from build123d import *

# Parameters (mm, degrees)
BOSS_EXTRUDE1_DEPTH = 2.5
SKETCH2_R           = 2
SKETCH2_R_2         = 1
CUT_EXTRUDE1_DEPTH  = 5
BOSS_EXTRUDE2_DEPTH = 13
SKETCH6_W           = 75
SKETCH6_H           = 9
BOSS_EXTRUDE3_DEPTH = 7
BOSS_EXTRUDE4_DEPTH = 10
SKETCH8_W           = 38.5
SKETCH8_H           = 0.01
BOSS_EXTRUDE5_DEPTH = 0.3


with BuildPart() as part:
    # Sketch1 → Boss-Extrude1 (new body)
    with BuildSketch(Plane(origin=(0, 0, 0), x_dir=(1, 0, 0), z_dir=(0, 1, 0))):
        with BuildLine():
            Line((-58.5, 47.5), (58.5, 47.5))
            Line((58.5, 47.5), (58.5, 25))
            ThreePointArc((58.5, 25), (56, 22.5), (58.5, 20))
            Line((58.5, 20), (58.5, -47.5))
            Line((58.5, -47.5), (-52.5, -47.5))
            Line((-52.5, -47.5), (-52.5, -2.5))
            Line((-52.5, -2.5), (-58.5, 5.5))
            Line((-58.5, 5.5), (-58.5, 20))
            ThreePointArc((-58.5, 20), (-56, 22.5), (-58.5, 25))
            Line((-58.5, 25), (-58.5, 47.5))
        make_face()
    extrude(amount=BOSS_EXTRUDE1_DEPTH)

    # Sketch2 → Cut-Extrude1 (cut)
    with BuildSketch(Plane(origin=(0, 2.5, 0), x_dir=(1, 0, 0), z_dir=(0, 1, 0))):
        with Locations(Location((-11.054054054, 6.409494198, 0), (0, 0, 270))):
            Circle(SKETCH2_R)
        with Locations(Location((-30, -32.5, 0), (0, 0, 270))):
            Circle(SKETCH2_R)
        with Locations(Location((38.5, -32.5, 0), (0, 0, 270))):
            Circle(SKETCH2_R)
        with Locations(Location((-42.5, -45.5, 0), (0, 0, 270))):
            Circle(SKETCH2_R_2)
        with Locations(Location((31.5, -45.5, 0), (0, 0, 270))):
            Circle(SKETCH2_R_2)
    extrude(amount=-CUT_EXTRUDE1_DEPTH, mode=Mode.SUBTRACT)

    # Sketch3 → Boss-Extrude2 (add)
    with BuildSketch(Plane(origin=(0, 2.5, 0), x_dir=(1, 0, 0), z_dir=(0, 1, 0))):
        Polygon((-26.5, 47.5), (-26.5, 30.5), (48.5, 30.5), (48.5, 47.5), (48.5, 51), (-26.5, 51), align=None)
    extrude(amount=BOSS_EXTRUDE2_DEPTH)

    # Sketch6 → Boss-Extrude3 (add)
    with BuildSketch(Plane(origin=(0, 2.5, 0), x_dir=(1, 0, 0), z_dir=(0, 1, 0))):
        with Locations((13, 24.5)):
            Rectangle(SKETCH6_W, SKETCH6_H)
    extrude(amount=BOSS_EXTRUDE3_DEPTH)

    # Sketch7 → Boss-Extrude4 (add)
    with BuildSketch(Plane(origin=(0, 2.5, 0), x_dir=(1, 0, 0), z_dir=(0, 1, 0))):
        Polygon((50.5, 47.5), (50.5, 35.5), (56.5, 35.5), (56.5, 47.5), (56.5, 50.5), (50.5, 50.5), align=None)
        Polygon((-29.5, 47.5), (-29.5, 35.5), (-38, 35.5), (-38, 47.5), (-38, 51), (-29.5, 51), align=None)
        Polygon((-41, 35.5), (-48, 35.5), (-48, 47.5), (-48, 51), (-41, 51), (-41, 47.5), align=None)
    extrude(amount=BOSS_EXTRUDE4_DEPTH)

    # Sketch8 → Boss-Extrude5 (add)
    with BuildSketch(Plane(origin=(0, 2.5, 0), x_dir=(1, 0, 0), z_dir=(0, 1, 0))):
        with Locations((-0.75, -45.495)):
            Rectangle(SKETCH8_W, SKETCH8_H)
    extrude(amount=BOSS_EXTRUDE5_DEPTH)


solid = part.part
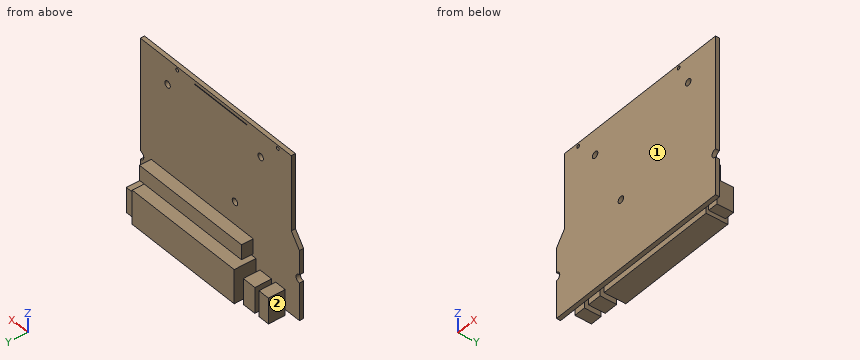
Design review of the part built by this model. Coordinates are the model's own, in mm. Face numbers are marked on the shaded views. A direction names the side the tool comes from. Give positions to 0.01 mm unless a question says otherwise; leave off trailing zeros. Order: outer loops, then holes, each group sorted by start corner. A loop starts at its lowest first (then second) coordinate and runs counter-clockwise, first axis right, second up.
1. Add section C-C, the plane y = 6.5. State the section outline as (x, z) points, then the cut area to 3 significant figures.
Solution:
outline: (-48, -51) - (-41, -51) - (-41, -35.5) - (-48, -35.5) - close; (-38, -51) - (-29.5, -51) - (-29.5, -35.5) - (-38, -35.5) - close; (-26.5, -51) - (48.5, -51) - (48.5, -30.5) - (-26.5, -30.5) - close; (-24.5, -29) - (50.5, -29) - (50.5, -20) - (-24.5, -20) - close; (50.5, -50.5) - (56.5, -50.5) - (56.5, -35.5) - (50.5, -35.5) - close
area: 2,540 mm2
2. Tool access review of the marked faces 1 and 2: name each direction out of +Z, -Z, +X, -X, +Y, -Y from which nothing blocks a thin tool from reaching the whole face with its end or side.
Solution:
face 1: +Z, -Z, +X, -X, -Y
face 2: +Z, -Z, -X, +Y
3. Add section B-B, the plane z = 32.5. State the section outline as (x, y) points.
Solution:
outline: (-52.5, 0) - (-32, 0) - (-32, 2.5) - (-52.5, 2.5) - close; (-28, 0) - (36.5, 0) - (36.5, 2.5) - (-28, 2.5) - close; (40.5, 0) - (58.5, 0) - (58.5, 2.5) - (40.5, 2.5) - close
4. To check wall thickness, follow L1, parallel to X at y = 7, z = -41.5; L2, parallel to Z at x = -1, y = 9.25; L3, parallel to X at y = 0.8, z = 45.5. State the ranges of each line that lie inside material, in increasing order.
Solution:
L1: x = -48 to -41, -38 to -29.5, -26.5 to 48.5, 50.5 to 56.5
L2: z = -51 to -30.5, -29 to -20
L3: x = -52.5 to -43.5, -41.5 to 30.5, 32.5 to 58.5
5. For pin 1 Ø5 at (x, y) = (-0.5, 10) entering from +Z; pin 2 Ø8 at (y, z) = (8.5, -46) entering from +X; pin 3 Ø3 at (y, z) = (1, 22.5) entering from -X, all flat-tipped, find the tip position at first contact; note any pin that passes through.
Solution:
pin 1: stops at z = -20
pin 2: stops at x = 56.5
pin 3: stops at x = -52.5
6. Add section A-A, the plane x = 38.5. State the section outline as (y, z) points.
Solution:
outline: (0, -47.5) - (2.5, -47.5) - (2.5, -51) - (15.5, -51) - (15.5, -30.5) - (2.5, -30.5) - (2.5, -29) - (9.5, -29) - (9.5, -20) - (2.5, -20) - (2.5, 30.5) - (0, 30.5) - close; (0, 34.5) - (2.5, 34.5) - (2.5, 47.5) - (0, 47.5) - close
